```python
from build123d import *

# Parameters (mm, degrees)
SKETCH1_R           = 1
BOSS_EXTRUDE1_DEPTH = 3
SKETCH2_W           = 50
SKETCH2_H           = 17
CUT_EXTRUDE1_DEPTH  = 177.568989461


with BuildPart() as part:
    # Sketch1 → Boss-Extrude1 (new body)
    with BuildSketch(Plane(origin=(0, 0, 0), x_dir=(1, 0, 0), z_dir=(0, 1, 0))):
        with BuildLine():
            Line((0, 0), (150.612084668, 12.621940938))
            ThreePointArc((150.612084668, 12.621940938), (166.192388155, 29.562556682), (150.612084668, 46.503172427))
            Line((150.612084668, 46.503172427), (0, 59.125113365))
            Line((0, 59.125113365), (-5, 59.562556682))
            Line((-5, 59.562556682), (-5, -0.437443318))
            Line((-5, -0.437443318), (0, 0))
        make_face()
        with Locations(Location((140, 38.754944838, 0), (0, 0, 270))):
            Circle(SKETCH1_R, mode=Mode.SUBTRACT)
        with Locations(Location((140, 20.370168527, 0), (0, 0, 270))):
            Circle(SKETCH1_R, mode=Mode.SUBTRACT)
        with Locations(Location((158.384776311, 20.370168527, 0), (0, 0, 270))):
            Circle(SKETCH1_R, mode=Mode.SUBTRACT)
        with Locations(Location((158.384776311, 38.754944838, 0), (0, 0, 270))):
            Circle(SKETCH1_R, mode=Mode.SUBTRACT)
    extrude(amount=BOSS_EXTRUDE1_DEPTH)

    # Sketch2 → Cut-Extrude1 (cut, through all)
    with BuildSketch(Plane(origin=(0, 3, 0), x_dir=(1, 0, 0), z_dir=(0, 1, 0))):
        with Locations((60, 29.562556682)):
            Rectangle(SKETCH2_W, SKETCH2_H)
    extrude(amount=-CUT_EXTRUDE1_DEPTH, mode=Mode.SUBTRACT)


solid = part.part
```
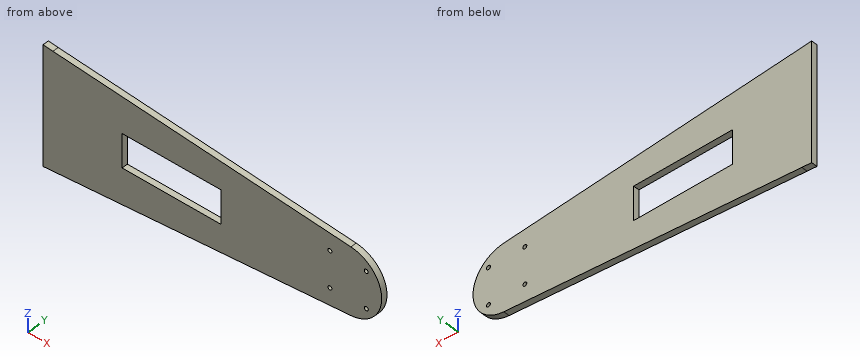
Work out the finished part from the listing and answer in its coordinate system (mm). Give positions to 0.01 mm unless a question says otherwise; leave off trailing zeros. Order: outer loops, then holes, each group sorted by start corner. A loop starts at its lowest first (then second) coordinate and runs counter-clockwise, first axis right, second up. Notation, with made-up numbers: (11.25, 59.5) - (39.25, 59.5) arc R25 ccw to (39.25, 77.5) - close; hole circle Ø1 at (80, -22.75). An arc over 180 degrees is marked (long way). One line per item, written item: value. Start each with the question number.
1. Section D-D, the plane z = -10 is taken. Write down the section's boundary in (x, y).
2. Section C-C, the plane y = 1.15 is taken. Write down the section's boundary in (x, z), then the cut area to 3 significant figures.
3. Section B-B, the plane z = -28 is taken. Write down the section's boundary in (x, y), then the cut area to 3 significant figures.
4. Section A-A, the plane x = 74 is taken. Write down the section's boundary in (y, z).
5. Consider line 1 (X direction, y = 2.15, z = -39.5); line 2 (Z direction, x = 140, y = 2.3); line 3 (X direction, y = 1.9, z = -30.5). Determine where each line is inside the solid, lowest interval first.
6. Each of these flat-tipped pins is pushed along its axis until it touches: pin 1 Ø1.5 at (y, z) = (1.5, -17) entering from +X; pin 2 Ø0.9 at (x, y) = (65.5, 1) entering from -Z; pin 3 Ø3 at (x, z) = (132.5, -50) entering from -Y (3 decimals); pin 4 Ø0.9 at (x, y) = (71, 2) entering from +Z. Where does it stop, or does it pass through?
Filled sheet:
1. outline: (-5, 0) - (119.33, 0) - (119.33, 3) - (-5, 3) - close
2. outline: (-5, -59.56) - (0, -59.13) - (150.61, -46.5) arc R17 ccw to (150.61, -12.62) - (0, 0) - (-5, 0.44) - close; hole (35, -38.06) - (85, -38.06) - (85, -21.06) - (35, -21.06) - close; hole circle Ø2 at (140, -38.75); hole circle Ø2 at (140, -20.37); hole circle Ø2 at (158.38, -38.75); hole circle Ø2 at (158.38, -20.37)
2. area: 6,840 mm²
3. outline: (-5, 0) - (35, 0) - (35, 3) - (-5, 3) - close; (85, 0) - (166.12, 0) - (166.12, 3) - (85, 3) - close
3. area: 363 mm²
4. outline: (0, -52.92) - (3, -52.92) - (3, -38.06) - (0, -38.06) - close; (0, -21.06) - (3, -21.06) - (3, -6.2) - (0, -6.2) - close
5. line 1: -5 to 139.33, 140.67 to 157.72, 159.05 to 162.99
5. line 2: -47.39 to -39.75, -37.75 to -21.37, -19.37 to -11.73
5. line 3: -5 to 35, 85 to 166.17
6. pin 1: x = 161.42
6. pin 2: z = -53.67
6. pin 3: through
6. pin 4: z = -5.91
